The figure shows three views and two pictorial views of one solid part (mm, origin at its lowest corner). Answer the questions. A direction names the side the tool comes from. Round coordinates to 2 decimals unless told otherwise and drop trailing zeros. Write each loop counter-clockwise with the first axis right and the second up, starting at its lowest first coordinate (ties: lowest second). Pieces come first, ordered by that corner, then holes.
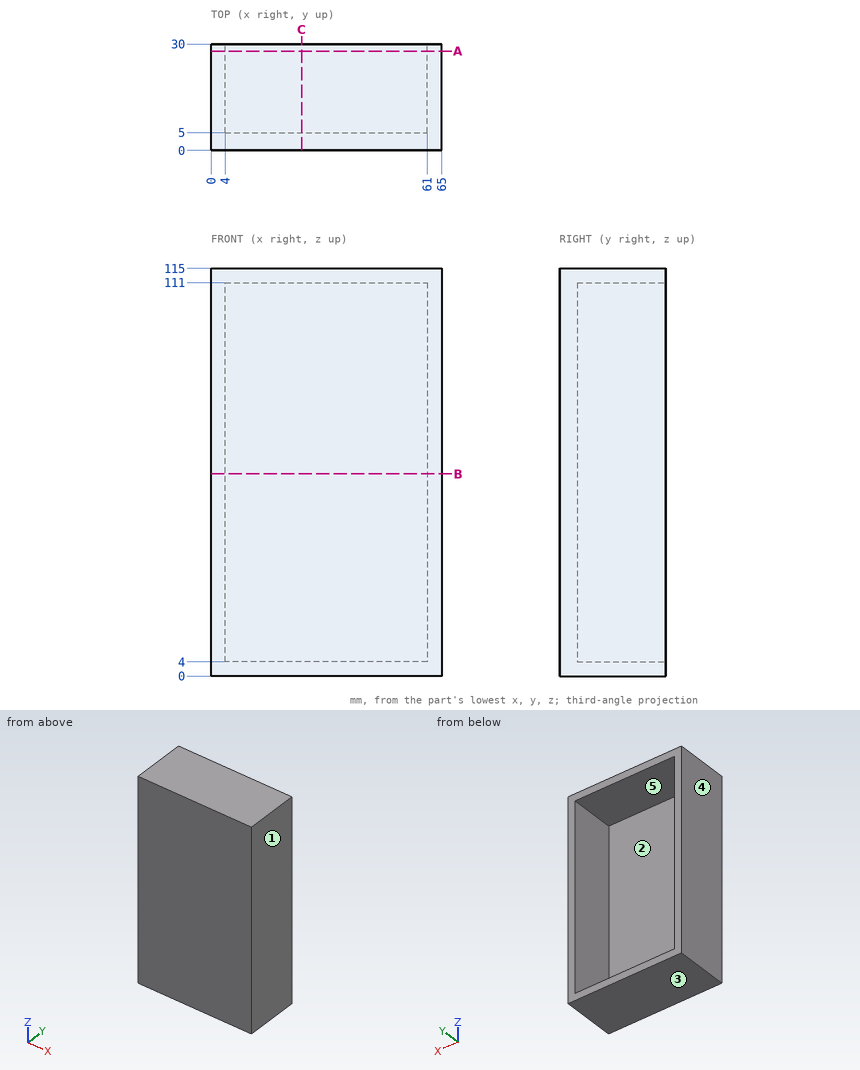
Q1. Section A-A (y = 28) is taken. Determine the outline of the cut face in (x, z), then the cut area to 3 significant figures.
Verdict:
outline: (0, 0) - (65, 0) - (65, 115) - (0, 115) - close; hole (4, 4) - (61, 4) - (61, 111) - (4, 111) - close
area: 1,380 mm2
Q2. Straight lines are drawn through the part: probe 1 along Z at (x, y) = (28, 21.75); probe 2 along X at (y, z) = (26, 59); probe 3 along Y at (x, z) = (47, 103). For each, find the intervals that lie inside material, in ascending order.
Verdict:
probe 1: z = 0 to 4, 111 to 115
probe 2: x = 0 to 4, 61 to 65
probe 3: y = 0 to 5
Q3. Section B-B (z = 57) is taken. Determine the outline of the cut face in (x, y).
Verdict:
outline: (0, 0) - (65, 0) - (65, 30) - (61, 30) - (61, 5) - (4, 5) - (4, 30) - (0, 30) - close
Q4. A flat-ended cylindrical pin translates along its axis: pin 1 Ø12 at (x, z) = (50, 40) entering from +Y. Find the tip coordinate at first contact, or state that the pin passes through.
Verdict:
pin 1: stops at y = 5
Q5. Section C-C (x = 25.5) is taken. Determine the outline of the cut face in (y, z), then the cut area to 3 significant figures.
Verdict:
outline: (0, 0) - (30, 0) - (30, 4) - (5, 4) - (5, 111) - (30, 111) - (30, 115) - (0, 115) - close
area: 775 mm2
Q6. Determine the mould class of the marked faces 3, 4 and 5 for opening direction X: pulls with the +X half, pulls with the -X half, needs draft (parallel to the pull), parting line crosses it, or undercut.
Verdict:
face 3: needs draft
face 4: pulls with the -X half
face 5: undercut
Q7. Which of the six approach directions +Z, -Z, +X, -X, +Y, -Y give full straight-line access (tool end or side, diameter ignored) to the marked faces 1 and 2?
Verdict:
face 1: +Z, -Z, +X, +Y, -Y
face 2: +Y
